Read the model definition and answer for the solid it produces. Units are mm, in the model's axes. A direction names the side the tool comes from. Coordinates: 2 decimals unless noted, no trailing zeros. Order: outer loops, then holes, each group sorted by start corner. A loop starts at its lowest first (then second) coordinate and runs counter-clockwise, first axis right, second up.
```python
from build123d import *

# Parameters (mm, degrees)
F2_SIZE        = 0.8128
F5_D           = 8.4836
F5_DEPTH       = 63.5
F5_CSINK_D     = 9.525
F5_CSINK_ANGLE = 60
F5_TIP         = 2.5487305738
F7_D           = 3.175
F7_DEPTH       = 38.1
F7_TIP         = 0.9538662327


# Not quite as in the source:
# - a fillet or chamfer that OpenCascade refuses, or shapes differently, is made with other operations: its cross-section is extruded or revolved along the edge and cut away or added


with BuildPart() as f1:
    # F0 (on Right) → F1 (revolve)
    with BuildSketch(Plane.YZ):
        Polygon((-177.8, 0), (0, 0), (0, 7.9375), (-19.05, 7.9375), (-19.05, 11.1125), (-31.75, 11.1125), (-31.75, 13.5128), (-44.45, 13.5128), (-44.45, 17.4625), (-152.4, 17.4625), (-152.4, 15.875), (-171.45, 15.875), (-180.975, 12.7), (-203.2, 12.7), (-203.2, 6.731), (-177.8, 6.731), align=None)
    revolve(axis=Axis((0, -88.9, 0), (0, -1, 0)))

    # F2
    f2_edges = [f1.edges().sort_by_distance(p)[0] for p in [
        (0, -203.2, -12.7),
        (0, -152.4, -17.4625),
        (0, -44.45, -17.4625),
        (0, -31.75, -13.5128),
        (0, 0, -7.9375),
    ]]
    chamfer(f2_edges, length=F2_SIZE)

    # F3: fillet of radius 3.175 on 1 edges, made by hand

    # F3_s1 → F3_t2 (revolve)
    with BuildSketch(Plane.YZ):
        with BuildLine():
            ThreePointArc((-41.2742745857, 13.5124), (-43.5064480149, 14.4289646435), (-44.4503999697, 16.6496950798))
            Line((-44.4503999697, 16.6496950798), (-44.7680125081, 16.6457880193))
            ThreePointArc((-44.7680125081, 16.6457880193), (-44.7676365685, 15.0812475399), (-44.7676365685, 13.5128))
            Line((-44.7676365685, 13.5128), (-44.45, 13.1951634315))
            ThreePointArc((-44.45, 13.1951634315), (-42.8621372928, 13.1951634315), (-41.2742745857, 13.1947634315))
            Line((-41.2742745857, 13.1947634315), (-41.2742745857, 13.5124))
        make_face()
    revolve(axis=Axis((0, -44.45, 0), (0, -1, 0)))

    # F5
    with Locations(Plane(origin=(0, 0, 0), x_dir=(-1, 0, 0), z_dir=(0, 1, 0))):
        with Locations((0, 0)):
            CounterSinkHole(F5_D / 2, F5_CSINK_D / 2, depth=F5_DEPTH, counter_sink_angle=F5_CSINK_ANGLE)
            with Locations((0, 0, -(F5_DEPTH + F5_TIP / 2))):  # 118° drill point
                Cone(0, F5_D / 2, F5_TIP, mode=Mode.SUBTRACT)

    # F7 (one way)
    with BuildSketch(Plane(origin=(0, 0, 0), x_dir=(0, 1, 0), z_dir=(-1, 0, 0))):
        with Locations((-36.915011704, 0)):
            Circle(F7_D / 2)
    extrude(amount=-F7_DEPTH, mode=Mode.SUBTRACT)
    with Locations(Plane(origin=(0, 0, 0), x_dir=(0, 1, 0), z_dir=(-1, 0, 0))):
        with Locations((-36.915011704, 0)):
            with Locations((0, 0, -(F7_DEPTH + F7_TIP / 2))):  # 118° drill point
                Cone(0, F7_D / 2, F7_TIP, mode=Mode.SUBTRACT)


solid = f1.part
```
1) Flat-ended cylindrical pins translate along their axes: pin 1 Ø2 at (y, z) = (-177, 4.5) entering from +X; pin 2 Ø4 at (y, z) = (-138.5, 3.5) entering from -X; pin 3 Ø8 at (x, z) = (0, 0) entering from -Y. Find the tip coordinate at first contact, or state that the pin passes through.
A:
pin 1: stops at x = 13.75
pin 2: stops at x = -17.4
pin 3: stops at y = -177.8
2) A cutting plane is placed at B-B, the plane y = -104. Determine the outline of the cut face in (x, z) (1 decimal), and give its area (3 significant figures).
A:
outline: circle Ø34.9 at (0, 0)
area: 958 mm2
3) A cutting plane is placed at A-A, the plane y = -190.5. Determine the outline of the cut face in (x, z), and give its area (3 significant figures).
A:
outline: circle Ø25.4 at (0, 0); hole circle Ø13.46 at (0, 0)
area: 364 mm2
4) Straight lines are drawn through the part: line 1 (Y direction, x = 7, z = 0); line 2 (Z direction, x = 0, y = -36.5); line 3 (Z direction, x = 0, y = -195). For each, find the intervals that lie inside material, in ascending order.
A:
line 1: y = -203.2 to -38.5, -35.33 to 0
line 2: z = -13.51 to -4.24, 4.24 to 13.51
line 3: z = -12.7 to -6.73, 6.73 to 12.7
5) Which of the six approach directions +Z, -Z, +X, -X, +Y, -Y give full straight-line access (tool end or side, diameter ignored) to faces 1 (the flat face through (5, -203.2, 5)), 2 (the cylindrical face through (-3.34, -25.49, 10.6)), 3 (the cylindrical face through (15.497, -162.058, -3.441))?
A:
face 1: +Z, -Z, +X, -X, -Y
face 2: +Y
face 3: -Y
